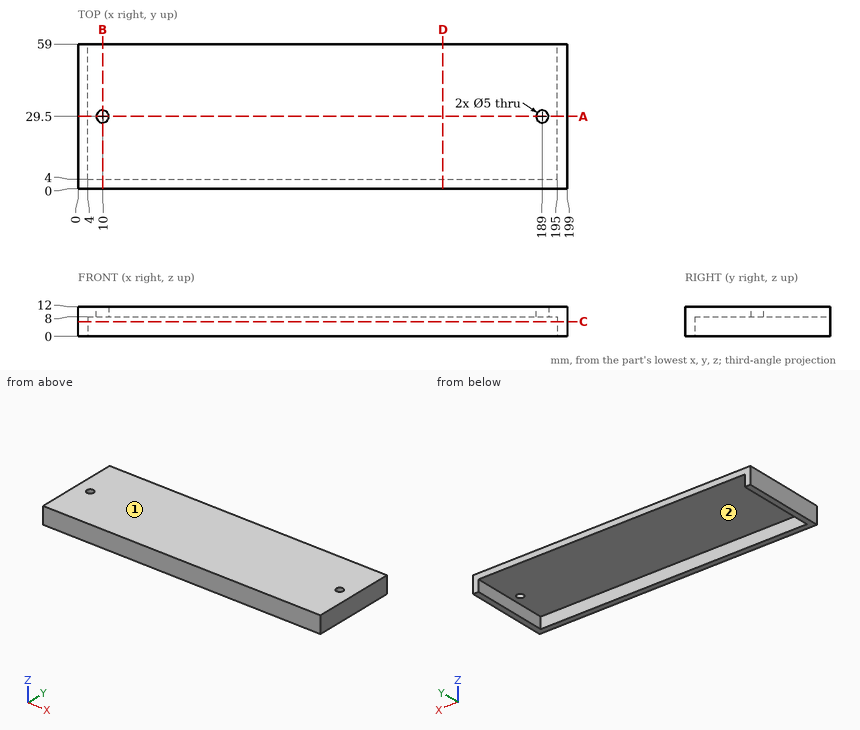
Geometry: see drawing. Coordinates: mm, zero at the bounding-box minimum. Give positions to 0.01 mm unless a question says otherwise; leave off trailing zeros. Loops run counter-clockwise (first coordinate to the right, second up) from the corner with the lowest first, then second, coordinate; pieces in that order, holes last. Notation, with made-up numbers: (29, 52.25) - (33, 52.25) arc R28 cw to (33, 87.25) - close; hole circle Ø11 at (9.25, 17). An arc over 180 degrees is marked (long way). One line per question, with ' | ' between items. Start each with the question number.
(1) Section query C-C on z = 6. Return loops of the section in (x, y).
(2) Contact query for flat-ended pins moving along their axis: pin 1 (2.5 mm diameter, centred on x = 122, z = 3.5, fed in from +Y); pin 2 (16.5 mm diameter, centred on x = 66, y = 41.5, fed in from -Z). Output: stop coordinate, or through.
(3) Section query B-B on x = 10. Return loops of the section in (y, z), then the cut area to 3 significant figures.
(4) Section query D-D on x = 148.5. Return loops of the section in (y, z), then the cut area to 3 significant figures.
(5) Ray query, line 1 (Y direction, x = 10, z = 9.1); line 2 (X direction, y = 17, z = 4.75); line 3 (Z direction, x = 158, y = 43). Return the intervals inside material, ascending. Write a range as from..to.
(6) Pull-direction query (X, two-part tool) for the marked faces 1 and 2; classes: released by +X, released by -X, zero draft, split by the parting line, or undercut.
(7) Section query A-A on y = 29.5. Return loops of the section in (x, z), then the cut area to 3 significant figures.
The answers:
1) outline: (0, 0) - (199, 0) - (199, 59) - (195, 59) - (195, 4) - (4, 4) - (4, 59) - (0, 59) - close
2) pin 1: y = 4 | pin 2: z = 8
3) outline: (0, 0) - (4, 0) - (4, 8) - (27, 8) - (27, 12) - (0, 12) - close; (32, 8) - (59, 8) - (59, 12) - (32, 12) - close | area: 248 mm2
4) outline: (0, 0) - (4, 0) - (4, 8) - (59, 8) - (59, 12) - (0, 12) - close | area: 268 mm2
5) line 1: 0..27, 32..59 | line 2: 0..4, 195..199 | line 3: 8..12
6) face 1: zero draft | face 2: undercut
7) outline: (0, 0) - (4, 0) - (4, 8) - (7.5, 8) - (7.5, 12) - (0, 12) - close; (12.5, 8) - (186.5, 8) - (186.5, 12) - (12.5, 12) - close; (191.5, 8) - (195, 8) - (195, 0) - (199, 0) - (199, 12) - (191.5, 12) - close | area: 820 mm2
